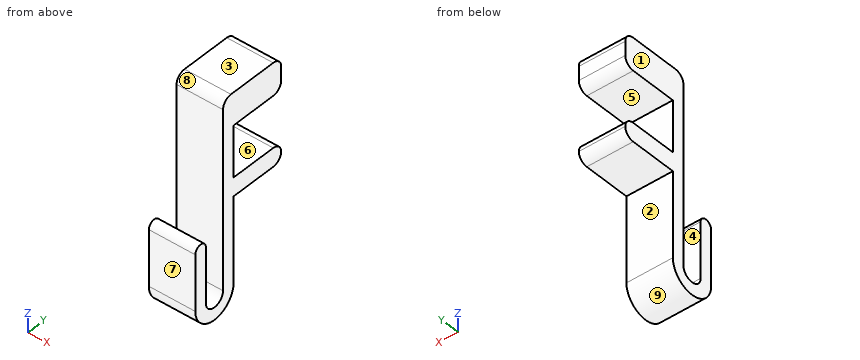
from build123d import *

# Parameters (mm, degrees)
F1_DEPTH = 15
F2_R     = 2.99999


# Not quite as in the source:
# - a fillet or chamfer is up to 0.001 mm smaller than in the source, because OpenCascade refuses the exact size


with BuildPart() as f1:
    # F0 (on Right) → F1 (new body)
    with BuildSketch(Plane.YZ):
        with BuildLine():
            Line((-18, 30.3650735612), (0, 30.3650735612))
            Line((0, 30.3650735612), (0, 40.8650735612))
            Line((0, 40.8650735612), (-22, 40.8650735612))
            Line((-22, 40.8650735612), (-22, -19.700880742))
            ThreePointArc((-22, -19.700880742), (-25.25, -22.950880742), (-28.5, -19.700880742))
            Line((-28.5, -19.700880742), (-28.5, -1.700880742))
            ThreePointArc((-28.5, -1.700880742), (-30.5, 0.299119258), (-32.5, -1.700880742))
            Line((-32.5, -1.700880742), (-32.5, -19.700880742))
            ThreePointArc((-32.5, -19.700880742), (-25.25, -26.950880742), (-18, -19.700880742))
            Line((-18, -19.700880742), (-18, 7.8150735612))
            Line((-18, 7.8150735612), (0, 7.8150735612))
            Line((0, 7.8150735612), (0, 13.8150735612))
            Line((0, 13.8150735612), (-18, 13.8150735612))
            Line((-18, 13.8150735612), (-18, 30.3650735612))
        make_face()
    extrude(amount=F1_DEPTH)

    # F2 (radius 3 in the source; OpenCascade refuses exactly that, so slightly less here)
    f2_edges = [f1.edges().sort_by_distance(p)[0] for p in [
        (7.5, 0, 30.365074),
        (7.5, 0, 13.815074),
        (7.5, 0, 40.865074),
        (7.5, 0, 7.815074),
        (7.5, -22, 40.865074),
    ]]
    fillet(f2_edges, radius=F2_R)


solid = f1.part
Geometry check sheet. Reference: the model listing, model coordinates, mm. Face numbers are marked on the shaded views. A direction names the side the tool comes from. Give positions to 0.01 mm unless a question says otherwise; leave off trailing zeros. Write each loop counter-clockwise with the first axis right and the second up, starting at its lowest first coordinate (ties: lowest second). Pieces come first, ordered by that corner, then holes. Notation, with made-up numbers: (86, 84.25) - (131, 84.25) arc R14 ccw to (131, 89.25) - close; hole circle Ø3 at (4, 34.25). An arc over 180 degrees is marked (long way). Put each result on its own line as item: value.
1. Sectioned sample at C-C, the plane z = 5. Enter the section's corners in (x, y).
Ans:
outline: (0, -22) - (15, -22) - (15, -18) - (0, -18) - close
2. Go/stop test with flat-tipped pins: pin 1 (10 mm diameter, centred on y = -12, z = 2.5, fed in from +X); pin 2 (7.5 mm diameter, centred on x = 9, z = 22, fed in from +Y); pin 3 (8 mm diameter, centred on x = 12, z = 16.5, fed in from -Y); pin 4 (7.5 mm diameter, centred on x = 9, y = -10.5, fed in from -Z). Record where each tip stops, or that it passes through.
Ans:
pin 1: passes through
pin 2: stops at y = -18
pin 3: stops at y = -22
pin 4: stops at z = 7.82
3. Sectioned sample at D-D, the plane y = -25.25. Enter the section's corners in (x, z).
Ans:
outline: (0, -26.95) - (15, -26.95) - (15, -22.95) - (0, -22.95) - close
4. Set-up check for the marked faces 1, 2, 3, 4 and 5: record each of +Z, -Z, +X, -X, +Y, -Y from which the full face is reachable in a straight line by a thin tool's end or side.
Ans:
face 1: +Z, -Z, -X, +Y, -Y
face 2: -Z, +X, -X, +Y
face 3: +Z, +X, -X, +Y, -Y
face 4: +Z, +X, -X
face 5: +X, -X, +Y
5. Thickness scan on line 1 (Y direction, x = 5.75, z = -15.5); line 2 (Z direction, x = 3.75, y = -17.5); line 3 (Y direction, x = 5.5, z = 21.5). Record the ranges inside material, lowest first.
Ans:
line 1: y = -32.5 to -28.5, -22 to -18
line 2: z = 7.82 to 13.82, 30.37 to 40.87
line 3: y = -22 to -18
6. Draft check along Z on the marked faces 6, 7, 8 and 9. Enter one of: +Z half, -Z half, draft (parallel to the pull), parting line (faces both ways), or undercut.
Ans:
face 6: undercut
face 7: draft
face 8: +Z half
face 9: -Z half
7. Sectioned sample at A-A, the plane z = -5.5. Enter the section's corners in (x, y).
Ans:
outline: (0, -32.5) - (15, -32.5) - (15, -28.5) - (0, -28.5) - close; (0, -22) - (15, -22) - (15, -18) - (0, -18) - close
